```python
from build123d import *

# Parameters (mm, degrees)
F0_W     = 16
F0_H     = 40
F1_DEPTH = 15
F2_R     = 6
F3_DEPTH = 16.001
F4_R     = 3
F5_DEPTH = 15.001
F6_SIZE  = 1


with BuildPart() as f1:
    # F0 (on Front) → F1 (new body)
    with BuildSketch(Plane.XZ):
        Rectangle(F0_W, F0_H)
    extrude(amount=F1_DEPTH)

    # F2 (on face) → F3 (cut, through all)
    with BuildSketch(Plane(origin=(-8, 0, 0), x_dir=(0, -1, 0), z_dir=(-1, 0, 0))):
        with Locations((-0.5, 0)):
            Circle(F2_R)
    extrude(amount=-F3_DEPTH, mode=Mode.SUBTRACT)

    # F4 (on Front) → F5 (cut, through all)
    with BuildSketch(Plane.XZ):
        with Locations((0, 13)):
            Circle(F4_R)
        with Locations((0, -13)):
            Circle(F4_R)
    extrude(amount=F5_DEPTH, mode=Mode.SUBTRACT)

    # F6
    f6_edges = [f1.edges().sort_by_distance(p)[0] for p in [
        (8, -7.5, 20),
        (-8, -7.5, 20),
        (8, -7.5, -20),
        (-8, -7.5, -20),
        (-8, -15, 0),
        (0, -15, -20),
        (8, -15, 0),
        (0, -15, 20),
    ]]
    chamfer(f6_edges, length=F6_SIZE)


solid = f1.part
```
Geometry: final body of the model. Coordinates: model frame, mm. Coordinates: 2 decimals unless noted, no trailing zeros. Write each loop counter-clockwise with the first axis right and the second up, starting at its lowest first coordinate (ties: lowest second). Pieces come first, ordered by that corner, then holes. Notation, with made-up numbers: M 4,39.5 L 38,39.5 A28 cw 38,66.5 Z; hole C 56.25,8 d10. An arc over 180 degrees is marked long. Use CSV: the item, a comma, the result in double quotes. Start each with the question number.
1. Cut plane C-C on z = 13. Return the cut outline in (x, y).
2. First-contact query: P1, Ø6, axis at x = -0.5, z = 15, coming from the -Y side; P2, Ø3.5, axis at x = 0, z = 13, coming from the +Y side. Flat tips, straight axial feed; report the tip coordinate or a pass-through.
3. Cut plane B-B on y = -10.75. Return the cut outline in (x, z), plus the area to 3 significant figures.
4. Mould query, pull axis Z, two halves, no side actions, for faces 1 (the face through (7.3, -14.4, -19.3)), 2 (the face through (-0.1, -5.5, -0.1)), 3 (the face through (7.3, -14.4, 19.3)). Classes: pulls with the +Z half, pulls with the -Z half, needs draft (parallel to the pull), parting line crosses it, or undercut.
5. Ray query, probe 1 along Z at (x, y) = (0, -9.5); probe 2 along X at (y, z) = (-7.5, 13); probe 3 along Z at (x, y) = (-1.75, -13.5). Return the intervals inside material, ascending.
6. Cut plane A-A on x = 0. Return the cut outline in (y, z).
7. Cut plane D-D on x = 4.75. Return the cut outline in (y, z), plus the area to 3 significant figures.
Entries:
1,outline,"M -8,-14 L -7,-15 L -3,-15 L -3,0 L -8,0 Z; M 3,-15 L 7,-15 L 8,-14 L 8,0 L 3,0 Z"
2,P1,"y = -15"
2,P2,"through"
3,outline,"M -8,-19 L -7,-20 L 7,-20 L 8,-19 L 8,19 L 7,20 L -7,20 L -8,19 Z; hole C 0,-13 d6; hole C 0,13 d6"
3,area,"581 mm²"
4,face 1,"pulls with the -Z half"
4,face 2,"undercut"
4,face 3,"pulls with the +Z half"
5,probe 1,"-20 to -16, -10 to 10, 16 to 20"
5,probe 2,"-8 to -3, 3 to 8"
5,probe 3,"-20 to -15.44, -10.56 to 10.56, 15.44 to 20"
6,outline,"M -15,-19 L -14,-20 L 0,-20 L 0,-16 L -15,-16 Z; M -15,-10 L 0,-10 L 0,-5.98 A6 cw 0,5.98 L 0,10 L -15,10 Z; M -15,16 L 0,16 L 0,20 L -14,20 L -15,19 Z"
7,outline,"M -15,-19 L -14,-20 L 0,-20 L 0,-5.98 A6 cw 0,5.98 L 0,20 L -14,20 L -15,19 Z"
7,area,"548 mm²"
